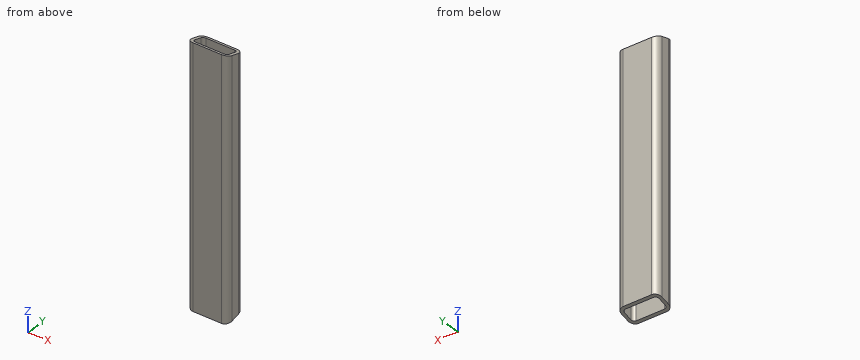
from build123d import *

# Parameters (mm, degrees)
EXTRUDE_1_DEPTH      = 126
EXTRUDE_1_DEPTH_BACK = 126
SHELL_1_T            = -3
CHAMFER_1_SIZE       = 5.358983849
CHAMFER_1_SIZE_2     = 20


with BuildPart() as part:
    # Эскиз1 → Бобышка-Вытянуть1 (new, two sides: drawn at the far end of the back side and taken through both)
    with BuildSketch(Plane.XY.offset(-EXTRUDE_1_DEPTH_BACK)):
        with BuildLine():
            Line((-14, 10), (14, 10))
            ThreePointArc((14, 10), (18.242640687, 8.242640687), (20, 4))
            Line((20, 4), (20, -4))
            ThreePointArc((20, -4), (18.242640687, -8.242640687), (14, -10))
            Line((14, -10), (-14, -10))
            ThreePointArc((-14, -10), (-18.242640687, -8.242640687), (-20, -4))
            Line((-20, -4), (-20, 4))
            ThreePointArc((-20, 4), (-18.242640687, 8.242640687), (-14, 10))
        make_face()
    extrude(amount=EXTRUDE_1_DEPTH + EXTRUDE_1_DEPTH_BACK)

    # Оболочка1
    shell_1_openings = [part.faces().sort_by_distance(p)[0] for p in [
        (0, 0, -126),
        (0, 0, 126),
    ]]
    offset(amount=SHELL_1_T, openings=shell_1_openings, kind=Kind.INTERSECTION)

    # Фаска1
    # the kernel refuses this chamfer: 20, 5.358983849 mm, written as the material it takes off along each edge
    with BuildSketch(Plane(origin=(-65.934431404, 10, -126), x_dir=(0, 0.13751244702128945, 0.9905000388259543), z_dir=(1, 0, 0))) as chamfer_1_piece_1:
        Polygon((CHAMFER_1_SIZE * 0.990500038756, CHAMFER_1_SIZE * 0.137512447012), (-CHAMFER_1_SIZE_2 * 0.137512447021, CHAMFER_1_SIZE_2 * 0.990500038826), (0, 0), align=None)
    extrude(amount=131.868862808, mode=Mode.SUBTRACT)
    with BuildSketch(Plane(origin=(-65.934431404, 10, 126), x_dir=(0, 0.13751244702128945, -0.9905000388259543), z_dir=(1, 0, 0))) as chamfer_1_piece_2:
        Polygon((CHAMFER_1_SIZE * 0.990500038756, -CHAMFER_1_SIZE * 0.137512447012), (-CHAMFER_1_SIZE_2 * 0.137512447021, -CHAMFER_1_SIZE_2 * 0.990500038826), (0, 0), align=None)
    extrude(amount=131.868862808, mode=Mode.SUBTRACT)


solid = part.part
Source: CAD feature listing. Evaluate the final solid. Frame: model axes, mm. Give positions to 0.01 mm unless a question says otherwise; leave off trailing zeros. Write each loop counter-clockwise with the first axis right and the second up, starting at its lowest first coordinate (ties: lowest second). Pieces come first, ordered by that corner, then holes. Notation, with made-up numbers: M 22.5,55 L 40.5,55 A12 ccw 40.5,73 Z; hole C -27.75,40.5 d8. An arc over 180 degrees is marked long. Answer as a JSON object with one key per item and string values.
Q1. Ray query, line 1 along Y through (x, z) = (4, 38.5); line 2 along X through (y, z) = (-3.75, -53.5); line 3 along Y through (x, z) = (15.5, 32). Return the intervals inside material, ascending.
Geometry check:
{"line 1": "y = -10 to -7, 7 to 10", "line 2": "x = -20 to -17, 17 to 20", "line 3": "y = -9.81 to -6.6, 6.6 to 9.81"}
Q2. Cut plane B-B, the plane z = -24.5. Return the cut outline in (x, y).
Geometry check:
{"outline": "M -20,-4 A6 ccw -14,-10 L 14,-10 A6 ccw 20,-4 L 20,4 A6 ccw 14,10 L -14,10 A6 ccw -20,4 Z; hole M -17,-4 A3 ccw -14,-7 L 14,-7 A3 ccw 17,-4 L 17,4 A3 ccw 14,7 L -14,7 A3 ccw -17,4 Z"}
Q3. Cut plane C-C, the plane y = 0.75. Return the cut outline in (x, z), then the cut area to 3 significant figures.
Geometry check:
{"outline": "M -20,-123.12 L -17,-123.12 L -17,123.12 L -20,123.12 Z; M 17,-123.12 L 20,-123.12 L 20,123.12 L 17,123.12 Z", "area": "1,480 mm^2"}
Q4. Contact query for flat-ended pins moving along their axis: P1, Ø5, axis at y = 7, z = 41.5, coming from the -X side; P2, Ø12, axis at x = -14, y = -3.5, coming from the -Z side. Output: stop coordinate, or through.
Geometry check:
{"P1": "stops at x = -19.98", "P2": "stops at z = -125.87"}
Q5. Cut plane A-A, the plane x = -6. Return the cut outline in (y, z), then the cut area to 3 significant figures.
Geometry check:
{"outline": "M -10,-126 L -7,-125.2 L -7,125.2 L -10,126 Z; M 7,-121.44 L 10,-120.64 L 10,120.64 L 7,121.44 Z", "area": "1,480 mm^2"}
